```python
from build123d import *

# Parameters (mm, degrees)
SKETCH_1_R          = 2.25
EXTRUDE_2_DEPTH     = 20
SKETCH_7_W          = 2.4
SKETCH_7_H          = 2.4
CUT_EXTRUDE_3_DEPTH = 2.5
SKETCH_9_R          = 3
EXTRUDE_4_DEPTH     = 1
SKETCH_10_W         = 4
SKETCH_10_H         = 4
EXTRUDE_5_DEPTH     = 2
FILLET_1_R          = 2


with BuildPart() as part:
    # 草图1 → 凸台-拉伸2 (new body)
    with BuildSketch(Plane.XY):
        Circle(SKETCH_1_R)
    extrude(amount=EXTRUDE_2_DEPTH)

    # 草图7 → 切除-拉伸3 (cut)
    with BuildSketch(Plane.XY):
        Rectangle(SKETCH_7_W, SKETCH_7_H)
    extrude(amount=CUT_EXTRUDE_3_DEPTH, mode=Mode.SUBTRACT)

    # 草图9 → 凸台-拉伸4 (add)
    with BuildSketch(Plane.XY.offset(20)):
        Circle(SKETCH_9_R)
    extrude(amount=EXTRUDE_4_DEPTH)

    # 草图10 → 凸台-拉伸5 (add)
    with BuildSketch(Plane.XY.offset(21)):
        Rectangle(SKETCH_10_W, SKETCH_10_H)
    extrude(amount=EXTRUDE_5_DEPTH)

    # 圆角1
    # the kernel refuses this fillet: 2 mm, written as the material it adds along each edge
    with BuildSketch(Plane(origin=(0, 0, 20), x_dir=(1, 0, 0), z_dir=(0, -1, 0))) as fillet_1_piece_1:
        with BuildLine():
            CenterArc((4.25, -1.5612495), FILLET_1_R, 128.682187453, 51.317812547)
            Line((2.25, -1.5612495), (2.21, -1.5612495))
            Line((2.21, -1.5612495), (2.21, 0))
            Line((2.21, 0), (2.25, 0.04))
            ThreePointArc((2.25, 0.04), (2.625, 0.04), (2.975, 0.03122499))
            Line((2.975, 0.03122499), (3, 0))
        make_face()
    revolve(axis=Axis((0, 0, 20), (0, 0, 1)))


solid = part.part
```
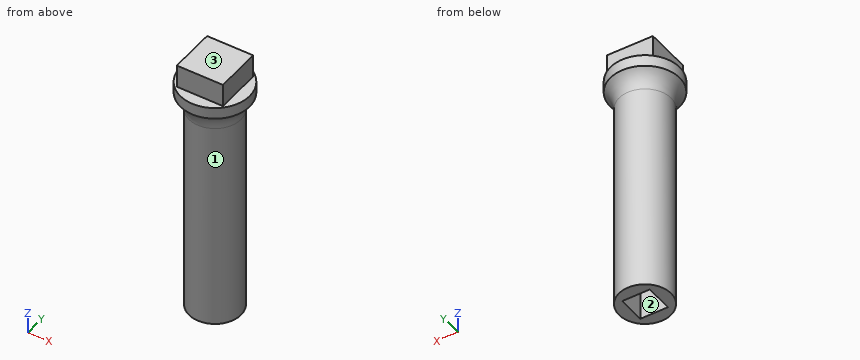
Verification items for the finished model (mm, model axes). Face numbers are marked on the shaded views. Round coordinates to 2 decimals unless told otherwise and drop trailing zeros. Write each loop counter-clockwise with the first axis right and the second up, starting at its lowest first coordinate (ties: lowest second). Pieces come first, ordered by that corner, then holes. Notation, with made-up numbers: (-27, 18) - (20, 18) arc R16 ccw to (20, 26) - close; hole circle Ø10 at (13.25, -34). An arc over 180 degrees is marked (long way). Answer as a JSON object with one key per item and string values. Group by question number.
Q1. Thickness scan on line 1 (Y direction, x = 0, z = 12.5); line 2 (Y direction, x = -0.5, z = 21.75); line 3 (Z direction, x = -0.5, y = 0.4). Record the ranges inside material, lowest first.
Q2. Mould release check, pull along X, two halves, no side actions. Record for the marked faces 1, 2 and 3: released by +X, released by -X, zero draft, split by the parting line, or undercut.
Q3. Go/stop test with flat-tipped pins: pin 1 Ø2 at (x, z) = (1, 15.5) entering from +Y; pin 2 Ø1.6 at (x, z) = (-1, 22) entering from -Y; pin 3 Ø1 at (y, z) = (2, 20) entering from +X. Record where each tip stops, or that it passes through.
Q4. Section check A-A, the plane x = 0. Enter the section's corners in (y, z), plus the area to 3 significant figures.
Q5. Section check C-C, the plane z = 10.75. Enter the section's corners in (x, y), plus the area to 3 significant figures.
Found:
{
 "1": {"line 1": "y = -2.25 to 2.25", "line 2": "y = -2 to 2", "line 3": "z = 2.5 to 23"},
 "2": {"face 1": "split by the parting line", "face 2": "undercut", "face 3": "zero draft"},
 "3": {"pin 1": "stops at y = 2.25", "pin 2": "stops at y = -2", "pin 3": "stops at x = 2.6"},
 "4": {"outline": "(-3, 20) arc R2 cw to (-2.25, 18.44) - (-2.25, 0) - (-1.2, 0) - (-1.2, 2.5) - (1.2, 2.5) - (1.2, 0) - (2.25, 0) - (2.25, 18.44) arc R2 cw to (3, 20) - (3, 21) - (2, 21) - (2, 23) - (-2, 23) - (-2, 21) - (-3, 21) - close", "area": "98.7 mm^2"},
 "5": {"outline": "circle Ø4.5 at (0, 0)", "area": "15.9 mm^2"}
}
